Source: CAD feature listing. Evaluate the final solid. Frame: model axes, mm. A direction names the side the tool comes from. Give positions to 0.01 mm unless a question says otherwise; leave off trailing zeros. Loops run counter-clockwise (first coordinate to the right, second up) from the corner with the lowest first, then second, coordinate; pieces in that order, holes last. Notation, with made-up numbers: (-20.5, -14.5) - (31.5, -14.5) arc R28 ccw to (31.5, 21.5) - close; hole circle Ø6 at (26.5, -8). An arc over 180 degrees is marked (long way). Put each result on its own line as item: value.
```python
from build123d import *

# Parameters (mm, degrees)
SKETCH1_R           = 1
BOSS_EXTRUDE1_DEPTH = 10


with BuildPart() as part:
    # Sketch1 → Boss-Extrude1 (new body)
    with BuildSketch(Plane.XY):
        Polygon((-8.5, 14.722431864), (-8.5, 30.907477288), (8.5, 30.907477288), (8.5, 14.722431864), (22.516660498, 6.629909152), (14.016660498, -8.092522712), (0, 0), (-14.016660498, -8.092522712), (-22.516660498, 6.629909152), align=None)
        with Locations((-7, 27.907477288)):
            Circle(SKETCH1_R, mode=Mode.SUBTRACT)
        with Locations((7, 27.907477288)):
            Circle(SKETCH1_R, mode=Mode.SUBTRACT)
        with Locations((-7, 21.907477288)):
            Circle(SKETCH1_R, mode=Mode.SUBTRACT)
        with Locations((7, 21.907477288)):
            Circle(SKETCH1_R, mode=Mode.SUBTRACT)
        with Locations((-16.624355653, 0)):
            Circle(SKETCH1_R, mode=Mode.SUBTRACT)
        with Locations((-4.5, 7)):
            Circle(SKETCH1_R, mode=Mode.SUBTRACT)
        with Locations((4.5, 7)):
            Circle(SKETCH1_R, mode=Mode.SUBTRACT)
        with Locations((16.624355653, 0)):
            Circle(SKETCH1_R, mode=Mode.SUBTRACT)
    extrude(amount=BOSS_EXTRUDE1_DEPTH)


solid = part.part
```
1) Mould query, pull axis X, two halves, no side actions, for faces 1 (the cylindrical face through (-7.13, 28.9, 4.93)), 2 (the flat face through (0, 7, 0)), 3 (the flat face through (-18.21, -0.83, 4.93)), 4 (the cylindrical face through (-4.63, 7.99, 4.93)). Classes: pulls with the +X half, pulls with the -X half, needs draft (parallel to the pull), parting line crosses it, or undercut.
Check result:
face 1: undercut
face 2: needs draft
face 3: pulls with the -X half
face 4: undercut
2) Access query for faces 5 (the cylindrical face through (6.87, 28.9, 4.93)), 6 (the flat face through (-6.91, -3.99, 4.93)), 7 (the flat face through (-8.5, 23, 5)), 8 (the flat face through (8.5, 23, 5)). Directions: +Z, -Z, +X, -X, +Y, -Y. A direction counts if a zero-diameter tool reaches every point of the face in a straight line with its end or side. Return the directions, or none.
Check result:
face 5: +Z, -Z
face 6: +Z, -Z, -Y
face 7: +Z, -Z, -X, +Y
face 8: +Z, -Z, +X, +Y
3) Section query A-A, the plane x = 4.5. Output: boundary loops of the cut face in (y, z).
Check result:
outline: (-2.6, 0) - (6, 0) - (6, 10) - (-2.6, 10) - close; (8, 0) - (30.91, 0) - (30.91, 10) - (8, 10) - close
4) Section query C-C, the plane x = -7. Output: boundary loops of the cut face in (y, z), plus the area to 3 significant figures.
Check result:
outline: (-4.04, 0) - (20.91, 0) - (20.91, 10) - (-4.04, 10) - close; (22.91, 0) - (26.91, 0) - (26.91, 10) - (22.91, 10) - close; (28.91, 0) - (30.91, 0) - (30.91, 10) - (28.91, 10) - close
area: 309 mm²
5) Section query B-B, the plane y = -4.5. Output: boundary loops of the cut face in (x, z).
Check result:
outline: (-16.09, 0) - (-7.79, 0) - (-7.79, 10) - (-16.09, 10) - close; (7.79, 0) - (16.09, 0) - (16.09, 10) - (7.79, 10) - close
6) Pin query (flat end, axial travel): P1, Ø3, axis at x = -16.62, y = 0, coming from the +Z side; P2, Ø1, axis at y = 23.5, z = 2.5, coming from the -X side; P3, Ø1.8, axis at x = 16.62, y = 0, coming from the -Z side; P4, Ø1, axis at x = 2, z = 2, coming from the -Y side. Return the tip coordinate at first contact, or that it passes through.
Check result:
P1: z = 10
P2: x = -8.5
P3: through
P4: y = -1.44
7) Material intervals for line 1 along X through (y, z) = (21.5, 0.5); line 2 along Y through (x, z) = (-7.5, 8.5); line 3 along X through (y, z) = (27, 6.5), sorted ascending. Write a range as [from, to].
Check result:
line 1: [-8.5, -7.91], [-6.09, 6.09], [7.91, 8.5]
line 2: [-4.33, 21.04], [22.77, 27.04], [28.77, 30.91]
line 3: [-8.5, -7.42], [-6.58, 6.58], [7.42, 8.5]
8) Section query D-D, the plane z = 6. State how many separate pieces and enclosed holes the cut face has, plus the area to 3 significant figures.
Check result:
separate pieces: 1
enclosed holes: 8
area: 925 mm²
